Can you work these out from the model? Positions are in its coordinate system, mm. A direction names the side the tool comes from. Give positions to 0.01 mm unless a question says otherwise; leave off trailing zeros. Order: outer loops, then holes, each group sorted by start corner. A loop starts at its lowest first (then second) coordinate and runs counter-clockwise, first axis right, second up. Notation, with made-up numbers: (77.25, 39.5) - (126.25, 39.5) arc R21 ccw to (126.25, 46.5) - close; hole circle Ø4 at (29, 35.5). An arc over 180 degrees is marked (long way). Use one line per item in the form item = value. Start each with the question number.
1) Which directions (+Z, -Z, +X, -X, +Y, -Y) give clear straight access to the entire face, cutting with the end or side of a thin tool? Please do faces 1 (the flat face through (-23.4, -23.8, 9.9)), 2 (the flat face through (16.6, -23.8, 9.9)), 3 (the flat face through (-0.75, 11, 8)).
2) Suppose I cut it at D-D, the plane z = 1.5. Write out the boundary of the cut face in (x, y).
3) Suppose I cut it at B-B, the plane x = 4.5. Write out the boundary of the cut face in (y, z) (3 decimals).
4) Please list where these lines run through material, in increasing order: probe 1 along X at (y, z) = (-27, 10) (3 decimals); probe 2 along X at (y, z) = (0, 6.25); probe 3 along Y at (x, z) = (6, 8).
5) Suppose I cut it at A-A, the plane y = 9. Write out the boundary of the cut face in (x, z), and give its area (3 significant figures).
6) For pin 1 (7.5 mm diameter, centred on y = 13.7, z = 10, fed in from -X); pin 2 (9 mm diameter, centred on y = 14, z = 14.5, fed in from +X); pin 3 (5 mm diameter, centred on x = 21, z = 12, fed in from +Y), each with a flat end and sliding along its axis, tell me the tip position at first contact or that it passes through.
7) We'd pull the mould along Z, two halves only. Please class faces 4 (the cylindrical face through (18.78, -27.5, 12.93)), 5 (the flat face through (0, -12, 20)), 6 (the flat face through (0, -12, 0)), 7 (the flat face through (8, 18.7, 10)): released by +Z, released by -Z, zero draft, split by the parting line, or undercut.
8) Suppose I cut it at C-C, the plane z = 12.25. Write out the boundary of the cut face in (x, y).
```python
from build123d import *

# Parameters (mm, degrees)
SALIENTE_EXTRUIR1_DEPTH    = 20
CROQUIS2_R                 = 3.175
CORTAR_EXTRUIR1_DEPTH      = 54.209491634
CORTAR_EXTRUIR2_DEPTH      = 55.586536802
CORTAR_EXTRUIR2_DEPTH_BACK = 55.586536802
CROQUIS3_R                 = 3.175


with BuildPart() as part:
    # Croquis1 → Saliente-Extruir1 (new body)
    with BuildSketch(Plane.XY):
        with BuildLine():
            Line((-15, 18.7), (-0.75, 18.7))
            Line((-0.75, 18.7), (-0.75, 7.361895136))
            ThreePointArc((-0.75, 7.361895136), (0, -7.4), (0.75, 7.361895136))
            Line((0.75, 7.361895136), (0.75, 18.7))
            Line((0.75, 18.7), (15, 18.7))
            Line((15, 18.7), (15, -23.8))
            Line((15, -23.8), (25, -23.8))
            Line((25, -23.8), (25, -31.3))
            Line((25, -31.3), (-25, -31.3))
            Line((-25, -31.3), (-25, -23.8))
            Line((-25, -23.8), (-15, -23.8))
            Line((-15, -23.8), (-15, 18.7))
        make_face()
    extrude(amount=SALIENTE_EXTRUIR1_DEPTH)

    # Croquis2 → Cortar-Extruir1 (cut, through all)
    with BuildSketch(Plane(origin=(0, -23.8, 0), x_dir=(1, 0, 0), z_dir=(0, 1, 0))):
        with Locations(Location((-20, -10, 0), (0, 0, 270))):
            Circle(CROQUIS2_R)
        with Locations(Location((20, -10, 0), (0, 0, 270))):
            Circle(CROQUIS2_R)
    extrude(amount=-CORTAR_EXTRUIR1_DEPTH, mode=Mode.SUBTRACT)

    # Croquis3 → Cortar-Extruir2 (cut, two sides: drawn at the far end of the back side and taken through both)
    with BuildSketch(Plane(origin=(15, 0, 0), x_dir=(0, 0, -1), z_dir=(1, 0, 0)).offset(-CORTAR_EXTRUIR2_DEPTH_BACK)):
        with Locations(Location((-10, 13.7, 0), (0, 0, 90))):
            Circle(CROQUIS3_R)
    extrude(amount=CORTAR_EXTRUIR2_DEPTH + CORTAR_EXTRUIR2_DEPTH_BACK, mode=Mode.SUBTRACT)


solid = part.part
```
Result sheet:
q1.face_1 = +Z, -Z, -X, +Y
q1.face_2 = +Z, -Z, +X, +Y
q1.face_3 = +Z, -Z, +Y
q2.outline = (-25, -31.3) - (25, -31.3) - (25, -23.8) - (15, -23.8) - (15, 18.7) - (0.75, 18.7) - (0.75, 7.36) arc R7.4 cw (long way) to (-0.75, 7.36) - (-0.75, 18.7) - (-15, 18.7) - (-15, -23.8) - (-25, -23.8) - close
q3.outline = (-31.3, 0) - (-5.875, 0) - (-5.875, 20) - (-31.3, 20) - close; (5.875, 0) - (18.7, 0) - (18.7, 20) - (5.875, 20) - close; hole circle Ø6.35 at (13.7, 10)
q4.probe_1 = -25 to -23.175, -16.825 to 16.825, 23.175 to 25
q4.probe_2 = -15 to -7.4, 7.4 to 15
q4.probe_3 = -31.3 to -4.33, 4.33 to 11.23, 16.17 to 18.7
q5.outline = (-15, 0) - (-0.75, 0) - (-0.75, 20) - (-15, 20) - close; (0.75, 0) - (15, 0) - (15, 20) - (0.75, 20) - close
q5.area = 570 mm²
q6.pin_1 = -15
q6.pin_2 = 15
q6.pin_3 = -23.8
q7.face_4 = undercut
q7.face_5 = released by +Z
q7.face_6 = released by -Z
q7.face_7 = zero draft
q8.outline = (-25, -31.3) - (-22.24, -31.3) - (-22.24, -23.8) - (-25, -23.8) - close; (-17.76, -31.3) - (17.76, -31.3) - (17.76, -23.8) - (15, -23.8) - (15, 11.46) - (0.75, 11.46) - (0.75, 7.36) arc R7.4 cw (long way) to (-0.75, 7.36) - (-0.75, 11.46) - (-15, 11.46) - (-15, -23.8) - (-17.76, -23.8) - close; (-15, 15.94) - (-0.75, 15.94) - (-0.75, 18.7) - (-15, 18.7) - close; (0.75, 15.94) - (15, 15.94) - (15, 18.7) - (0.75, 18.7) - close; (22.24, -31.3) - (25, -31.3) - (25, -23.8) - (22.24, -23.8) - close
